from build123d import *

# Parameters (mm, degrees)
SKETCH_1_R               = 17.5
EXTRUDE_1_DEPTH          = 4
SKETCH_2_R               = 8
SKETCH_2_R_2             = 4
EXTRUDE_2_DEPTH          = 15
CUT_EXTRUDE_1_REACH      = 33.201
CUT_EXTRUDE_1_END_RADIUS = 8
SKETCH_3_R               = 2
FILLET_1_R               = 1
SKETCH_4_R               = 2
CUT_EXTRUDE_2_DEPTH      = 15


with BuildPart() as part:
    # 草图1 → 凸台-拉伸1 (new body)
    with BuildSketch(Plane(origin=(0, 0, 0), x_dir=(1, 0, 0), z_dir=(0, 1, 0))):
        with Locations(Location((0, 0, 0), (0, 0, 270))):
            Circle(SKETCH_1_R)
    extrude(amount=EXTRUDE_1_DEPTH)

    # 草图2 → 凸台-拉伸2 (add)
    with BuildSketch(Plane(origin=(0, 4, 0), x_dir=(1, 0, 0), z_dir=(0, 1, 0))):
        with Locations(Location((0, 0, 0), (0, 0, 270))):
            Circle(SKETCH_2_R)
        with Locations(Location((0, 0, 0), (0, 0, 270))):
            Circle(SKETCH_2_R_2, mode=Mode.SUBTRACT)
    extrude(amount=EXTRUDE_2_DEPTH)

    # 切除-拉伸1: up to this cylinder (the profile starts inside it)
    cut_extrude_1_end = Plane(origin=(0, 12, 0), z_dir=(0, -1, 0)) * Cylinder(CUT_EXTRUDE_1_END_RADIUS, 83.402, mode=Mode.PRIVATE)
    # 草图3 → 切除-拉伸1 (cut, up to the surface)
    with BuildSketch(Plane.XY, mode=Mode.PRIVATE) as cut_extrude_1_sk1:
        with Locations((0, 12)):
            Circle(SKETCH_3_R)
    cut_extrude_1_tool1 = extrude(cut_extrude_1_sk1.sketch, amount=-CUT_EXTRUDE_1_REACH, mode=Mode.PRIVATE) & cut_extrude_1_end
    add(cut_extrude_1_tool1.solids().sort_by_distance((0, 12, 0))[0], mode=Mode.SUBTRACT)

    # 圆角1
    fillet_1_edges = [part.edges().sort_by_distance(p)[0] for p in [
        (0, 0, -17.5),
        (0, 4, -17.5),
        (0, 19, -8),
    ]]
    fillet(fillet_1_edges, radius=FILLET_1_R)

    # 草图4 → 切除-拉伸2 (cut)
    with BuildSketch(Plane(origin=(0, 4, 0), x_dir=(1, 0, 0), z_dir=(0, 1, 0))):
        with Locations(Location((-13, 0, 0), (0, 0, 270))):
            Circle(SKETCH_4_R)
        with Locations(Location((0, -13, 0), (0, 0, 270))):
            Circle(SKETCH_4_R)
        with Locations(Location((0, 13, 0), (0, 0, 270))):
            Circle(SKETCH_4_R)
        with Locations(Location((13, 0, 0), (0, 0, 270))):
            Circle(SKETCH_4_R)
    extrude(amount=-CUT_EXTRUDE_2_DEPTH, mode=Mode.SUBTRACT)


solid = part.part
Design review of the part built by this model. Coordinates are the model's own, in mm. A direction names the side the tool comes from. Coordinates: 2 decimals unless noted, no trailing zeros. Loops run counter-clockwise (first coordinate to the right, second up) from the corner with the lowest first, then second, coordinate; pieces in that order, holes last. Notation, with made-up numbers: M 42.5,-14.75 L 49.5,-14.75 A27 ccw 49.5,15.25 Z; hole C -28.5,-10 d11. An arc over 180 degrees is marked long. Answer as CSV lines item,"result".
Item 1: For probe 1 along Z at (x, y) = (0, 7.5); probe 2 along Y at (x, z) = (2.5, 14); probe 3 along X at (y, z) = (12, -4.45), list the stretches that pass through material, from the lowest coordinate up.
Answer list:
probe 1,"-8 to -4, 4 to 8"
probe 2,"0 to 4"
probe 3,"-6.65 to -2, 2 to 6.65"
Item 2: Add section C-C on z = 0. State the section outline as (x, y) points.
Answer list:
outline,"M -17.5,1 A1 ccw -16.5,0 L -15,0 L -15,4 L -16.5,4 A1 ccw -17.5,3 Z; M -11,0 L 11,0 L 11,4 L 8,4 L 8,18 A1 ccw 7,19 L 4,19 L 4,4 L -4,4 L -4,19 L -7,19 A1 ccw -8,18 L -8,4 L -11,4 Z; M 15,0 L 16.5,0 A1 ccw 17.5,1 L 17.5,3 A1 ccw 16.5,4 L 15,4 Z"
Item 3: Add section A-A on x = 0. Count the separate pieces of the cut face and the enclosed holes in it, plus the area to 3 significant figures.
Answer list:
separate pieces,"4"
enclosed holes,"0"
area,"211 mm²"
Item 4: Add section D-D on y = 7.75. State the section outline as (x, z) points.
Answer list:
outline,"C 0,0 d16; hole C 0,0 d8"
Item 5: For P1, Ø2.5, axis at x = 0, y = 12, coming from the +Z side; P2, Ø6, axis at y = 8.5, z = 0.5, coming from the +X side; P3, Ø6.5, axis at x = 13, z = 0, coming from the +Y side; P4, Ø2.5, axis at x = -13, z = 0, coming from the +Y side, all flat-tipped, find the tip position at first contact; note any pin that passes through.
Answer list:
P1,"z = 8"
P2,"x = 8"
P3,"y = 4"
P4,"through"
Item 6: Machinability: for faces 1 (the face through (-3.06, 10.9, 7.39)), 2 (the face through (0, 10, -6)), 3 (the face through (15, 2, 0)), which of the approach directions +Z, -Z, +X, -X, +Y, -Y give a long, thin tool a straight path to every point of the face, cutting with its end or side? Answer none if there is none.
Answer list:
face 1,"+Y"
face 2,"-Z"
face 3,"+Y, -Y"
Item 7: The part is to be moulded in two halves that separate along Z. For faces 4 (the face through (-3, 19, 3)), 5 (the face through (0, 4, 0)), 6 (the face through (-10.648, 1.986, -13.887)), say which applies: pulls with the +Z half, pulls with the -Z half, needs draft (parallel to the pull), parting line crosses it, or undercut.
Answer list:
face 4,"needs draft"
face 5,"undercut"
face 6,"parting line crosses it"
Item 8: Add section B-B on y = 1.5. State the section outline as (x, z) points, plus the area to 3 significant figures.
Answer list:
outline,"C 0,0 d35; hole C -13,0 d4; hole C 0,-13 d4; hole C 0,13 d4; hole C 13,0 d4"
area,"912 mm²"
